The figure shows three views and two pictorial views of one solid part (mm, origin at its lowest corner). Answer the questions. A direction names the side the tool comes from. Round coordinates to 2 decimals unless told otherwise and drop trailing zeros. Write each loop counter-clockwise with the first axis right and the second up, starting at its lowest first coordinate (ties: lowest second). Pieces come first, ordered by that corner, then holes. Notation, with made-up numbers: M 16.5,22 L 58.5,22 A17 cw 58.5,29 Z; hole C -6.5,61 d6. An arc over 180 degrees is marked long. One line per item, written item: value. Start each with the question number.
Q1. Given pin 1 Ø6 at (x, y) = (43, 6) entering from +Z; pin 2 Ø5 at (y, z) = (25.5, 18.5) entering from -X; pin 3 Ø2 at (y, z) = (14.5, 12) entering from -X, each flat-ended and moving along its own axis, determine where each tip first touches the part or whether it passes through.
Q2. A tool of negligible diameter and unlimited length cuts with its end or side. For the marked faces 1 and 2, from which of +Z, -Z, +X, -X, +Y, -Y can it reach the whole face along a straight path? Write none if from no direction.
Q3. Find section B-B (y = 27). Write down the section's boundary in (x, z).
Q4. Find section D-D (y = 10). Write down the section's boundary in (x, z).
Q5. Find section C-C (y = 20). Write down the section's boundary in (x, z).
Q6. Find section A-A (x = 6). Write down the section's boundary in (y, z).
Q7. Consider probe 1 along Y at (x, z) = (6, 1.15); probe 2 along Z at (x, y) = (26.5, 31.5); probe 3 along Z at (x, y) = (51.5, 32.5) (1 decimal). Determine where each line is inside the solid, lowest interval first.
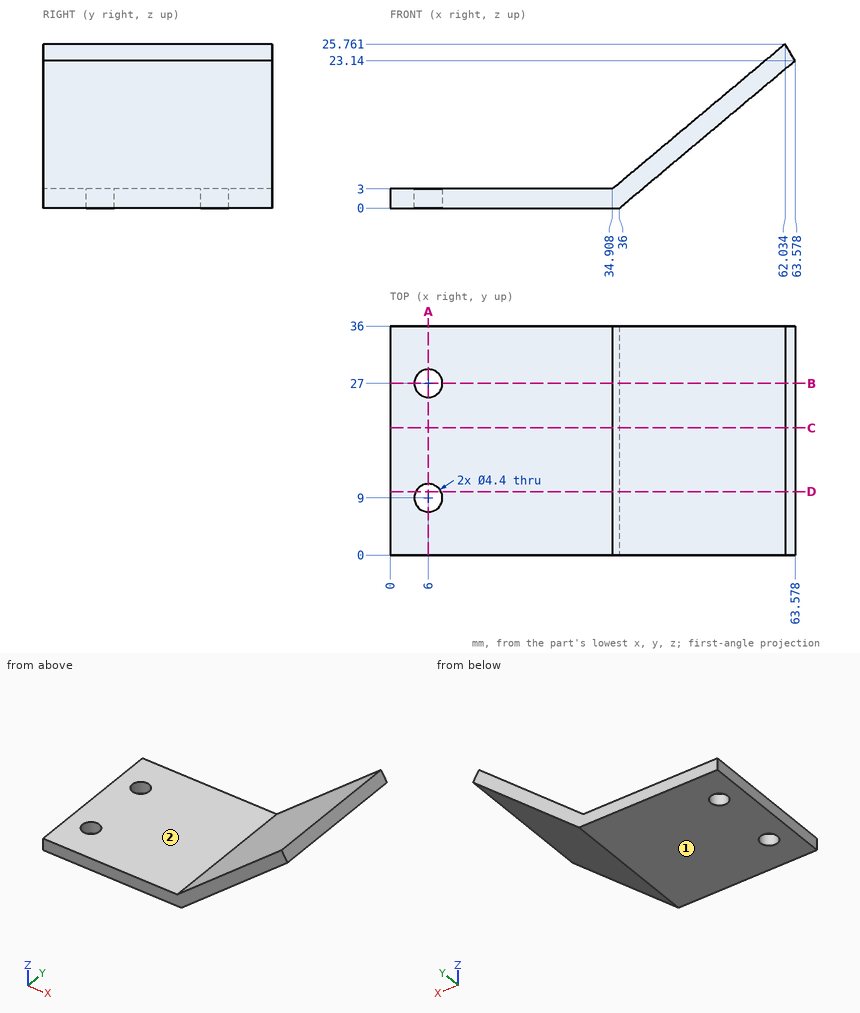
The answers:
1. pin 1: z = 12.31
1. pin 2: x = 50.4
1. pin 3: x = 44.44
2. face 1: -Z, +X, -X, +Y, -Y
2. face 2: +Z, -X, +Y, -Y
3. outline: M 0,0 L 3.8,0 L 3.8,3 L 0,3 Z; M 8.2,0 L 36,0 L 63.58,23.14 L 62.03,25.76 L 34.91,3 L 8.2,3 Z
4. outline: M 0,0 L 4.04,0 L 4.04,3 L 0,3 Z; M 7.96,0 L 36,0 L 63.58,23.14 L 62.03,25.76 L 34.91,3 L 7.96,3 Z
5. outline: M 0,0 L 36,0 L 63.58,23.14 L 62.03,25.76 L 34.91,3 L 0,3 Z
6. outline: M 0,0 L 6.8,0 L 6.8,3 L 0,3 Z; M 11.2,0 L 24.8,0 L 24.8,3 L 11.2,3 Z; M 29.2,0 L 36,0 L 36,3 L 29.2,3 Z
7. probe 1: 0 to 6.8, 11.2 to 24.8, 29.2 to 36
7. probe 2: 0 to 3
7. probe 3: 13 to 16.9
